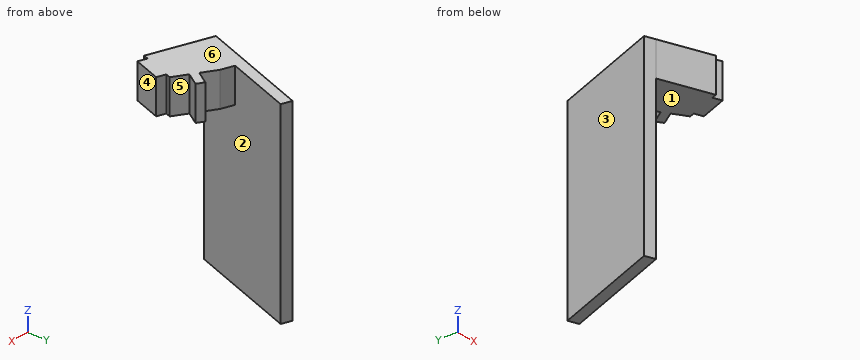
```python
from build123d import *

# Parameters (mm, degrees)
SKETCH1_W      = 203.2
SKETCH1_H      = 101.6
EXTRUDE1_DEPTH = 50.8
EXTRUDE2_DEPTH = 16.51
SKETCH23_W     = 203.2
SKETCH23_H     = 50.8
EXTRUDE3_DEPTH = 508
SKETCH24_W     = 16.51
SKETCH24_H     = 23.273283323
EXTRUDE6_DEPTH = 5.08


with BuildPart() as part:
    # Sketch1 → Extrude1 (new body)
    with BuildSketch(Plane.XY):
        with Locations((101.6, 50.8)):
            Rectangle(SKETCH1_W, SKETCH1_H)
    extrude(amount=EXTRUDE1_DEPTH)

    # Sketch21 → Extrude2 (add)
    with BuildSketch(Plane.XY.offset(50.8)):
        Polygon((10.680914086, 39.466921448), (16.647962228, 37.295093538), (23.464694461, 32.952356157), (27.558917476, 39.378998974), (30.772238885, 37.331887466), (26.678015869, 30.905244649), (33.104658686, 26.811021633), (32.238976379, 24.432579042), (36.293520259, 22.947359397), (31.515498857, 9.819853485), (27.43078785, 11.306566707), (26.589174956, 8.909877207), (2.720982388, 17.597188848), align=None)
    extrude(amount=EXTRUDE2_DEPTH)

    # Sketch23 → Extrude3 (cut)
    with BuildSketch(Plane.XZ):
        with Locations((101.6, 25.4)):
            Rectangle(SKETCH23_W, SKETCH23_H)
    extrude(amount=-EXTRUDE3_DEPTH, mode=Mode.SUBTRACT)

    # Sketch24 → Extrude6 (add)
    with BuildSketch(Plane(origin=(-3.252939565, 1.183973176, 0), x_dir=(0, 0, 1), z_dir=(-0.9396926207859065, 0.3420201433256742, 0))):
        Polygon((-25.295320048, 17.466579293), (50.8, 17.466579293), (50.8, 40.739862616), (67.31, 40.739862616), (67.31, 74.721559979), (50.8, 74.721559979), (-25.295320048, 74.721559979), align=None)
        with Locations((59.055, 29.103220955)):
            Rectangle(SKETCH24_W, SKETCH24_H)
    extrude(amount=EXTRUDE6_DEPTH)


solid = part.part
```
The listing builds one solid part. Answer for the finished solid, in the listing's coordinates (mm). Face numbers are marked on the shaded views. A direction names the side the tool comes from. Coordinates: 2 decimals unless noted, no trailing zeros. Write each loop counter-clockwise with the first axis right and the second up, starting at its lowest first coordinate (ties: lowest second). Pieces come first, ordered by that corner, then holes. Notation, with made-up numbers: M 2.25,22.5 L 44.25,22.5 A23 ccw 44.25,31.5 Z; hole C -7,10.25 d2. An arc over 180 degrees is marked long. Use a Markdown table: item, result. Add a question column.
1. For a pull along Y with two mould halves and no side action, classify the marked faces 3, 4, 5 and 6 as +Y half, -Y half, draft (parallel to the pull), parting line (faces both ways), or undercut.
2. Which of the six approach directions +Z, -Z, +X, -X, +Y, -Y give full straight-line access (tool end or side, diameter ignored) to the marked faces 1 and 2?
3. Straight lines are drawn through the part: line 1 along Z through (x, y) = (23, 30); line 2 along X through (y, z) = (51.5, 24); line 3 along X through (y, z) = (66, 16). For each, find the intervals that lie inside material, in ascending order. Write a range as [from, to].
4. Section C-C (z = 28) is taken. Give the vertices of the cut face in (x, y).
5. Section A-A (y = 35) is taken. Give the vertices of the cut face in (x, z), plus the area to 3 significant figures.
6. Section B-B (x = 15.5) is taken. Give the vertices of the cut face in (y, z).
7. Section D-D (y = 20.5) is taken. Give the vertices of the cut face in (x, z), plus the area to 3 significant figures.
8. Given P1, Ø3, axis at y = 24.5, z = 22, coming from the -X side; P2, Ø5, axis at y = 43, z = 23.5, coming from the +X side; P3, Ø12, axis at y = 62.5, z = 47.5, coming from the -X side, each flat-ended and moving along its own axis, determine where each tip first touches the part or whether it passes through.
Data:
| question | item | result |
|---|---|---|
| 1 | face 3 | +Y half |
| 1 | face 4 | -Y half |
| 1 | face 5 | undercut |
| 1 | face 6 | draft |
| 2 | face 1 | -Z, +X, -Y |
| 2 | face 2 | -Z, +X |
| 3 | line 1 | z = [50.8, 67.31] |
| 3 | line 2 | x = [9.65, 15.06] |
| 3 | line 3 | x = [14.93, 20.34] |
| 4 | outline | M -2.05,19.33 L 2.72,17.6 L 22.3,71.4 L 17.53,73.14 Z |
| 5 | outline | M 3.65,-25.3 L 9.06,-25.3 L 9.06,50.8 L 20.25,50.8 L 20.25,67.31 L 3.65,67.31 Z; M 24.77,50.8 L 29.29,50.8 L 29.29,67.31 L 24.77,67.31 Z |
| 5 | area | 760 mm2 |
| 6 | outline | M 12.95,50.8 L 37.71,50.8 L 37.71,67.31 L 12.95,67.31 Z; M 52.71,-25.3 L 67.56,-25.3 L 67.56,67.31 L 52.71,67.31 Z |
| 7 | outline | M -1.63,-25.3 L 3.78,-25.3 L 3.78,50.8 L 35.4,50.8 L 35.4,67.31 L -1.63,67.31 Z |
| 7 | area | 1,020 mm2 |
| 8 | P1 | stops at x = -0.72 |
| 8 | P2 | stops at x = 12.88 |
| 8 | P3 | stops at x = 11.47 |
